Design review of the part built by this model. Coordinates are the model's own, in mm. A direction names the side the tool comes from. Give positions to 0.01 mm unless a question says otherwise; leave off trailing zeros. Loops run counter-clockwise (first coordinate to the right, second up) from the corner with the lowest first, then second, coordinate; pieces in that order, holes last.
from build123d import *
from build123d.topology import SkipClean

# Parameters (mm, degrees)
BOSS_EXTRUDE1_DEPTH      = 15
CHAMFER1_SIZE            = 3.2
LPATTERN1_COUNT          = 2
LPATTERN1_PITCH          = 41.5
SKETCH4_W                = 5.3
SKETCH4_H                = 12.8
CUT_EXTRUDE1_DEPTH       = 81.375680401
SKETCH5_W                = 26.8
SKETCH5_H                = 15.8
CUT_EXTRUDE2_DEPTH       = 3.5
CUT_EXTRUDE_THIN11_REACH = 81.437
SKETCH6_W                = 26
SKETCH6_H                = 1.6


with BuildPart() as part:
    # Sketch1 → Boss-Extrude1 (new, symmetric)
    with BuildSketch(Plane(origin=(0, 0, 0), x_dir=(0, 0, -1), z_dir=(1, 0, 0))):
        Polygon((0, 0), (12, 3), (23.32165913, 12.5), (31.5, 12.5), (39.819620609, 6), (74, 6), (77, 3.65614312), (77, -3.157724852), (70, -11.5), (16, -11.5), (13.31488118, -8.3), (4.2, -4.6), align=None)
        Polygon((16.321122645, 3.753956381), (24.122393645, 10.3), (30.742479251, 10.3), (39.121033004, 3.753956381), align=None, mode=Mode.SUBTRACT)
    extrude(amount=BOSS_EXTRUDE1_DEPTH, both=True)

    # Chamfer1
    chamfer1_edges = [part.edges().sort_by_distance(p)[0] for p in [
        (-15, -11.5, -43),
        (15, -11.5, -43),
    ]]
    chamfer(chamfer1_edges, length=CHAMFER1_SIZE)

    # Sketch2 → Cut-Revolve1 (revolve, cut)
    with BuildSketch(Plane.XY.offset(-22.3), mode=Mode.PRIVATE) as cut_revolve1_sk:
        Polygon((15, 2.4), (10.15, 2.4), (3.75, -4), (0, -4), (0, -6.7), (15, -6.7), align=None)
    cut_revolve1 = revolve(cut_revolve1_sk.sketch.rotate(Axis((0, -6.7, -22.3), (-1, 0, 0)), 90), axis=Axis((0, -6.7, -22.3), (-1, 0, 0)), mode=Mode.SUBTRACT)

    # Mirror1: Cut-Revolve1 across plane
    add(cut_revolve1.mirror(Plane(origin=(0, 0, 0), x_dir=(0, 0, 1), z_dir=(1, 0, 0))), mode=Mode.SUBTRACT)

    # LPattern1: Cut-Revolve1 ×2
    with Locations(*[(0, 0, -i * LPATTERN1_PITCH) for i in range(1, LPATTERN1_COUNT)]):
        add(cut_revolve1, mode=Mode.SUBTRACT)

    # Mirror2 copy 1 sketch → Mirror2 copy 1 (revolve, cut)
    with BuildSketch(Plane(origin=(0, 0, -63.8), x_dir=(-1, 0, 0), z_dir=(0, 0, 1))):
        Polygon((15, -2.4), (10.15, -2.4), (3.75, 4), (0, 4), (0, 6.7), (15, 6.7), align=None)
    revolve(axis=Axis((0, -6.7, -63.8), (-1, 0, 0)), mode=Mode.SUBTRACT)

    # Mirror2 copy 2 sketch → Mirror2 copy 2 (revolve, cut)
    with SkipClean():  # the faces are left unmerged after this step: merging them gives an invalid solid
        with BuildSketch(Plane(origin=(0, 0, -22.3), x_dir=(-1, 0, 0), z_dir=(0, 0, 1))):
            Polygon((15, -2.4), (10.15, -2.4), (3.75, 4), (0, 4), (0, 6.7), (15, 6.7), align=None)
        revolve(axis=Axis((0, -6.7, -22.3), (-1, 0, 0)), mode=Mode.SUBTRACT)

    # Sketch4 → Cut-Extrude1 (cut, through all)
    with BuildSketch(Plane(origin=(0, 6, 0), x_dir=(1, 0, 0), z_dir=(0, 1, 0))):
        with Locations((6.85, 48.219620609)):
            Rectangle(SKETCH4_W, SKETCH4_H)
    cut_extrude1 = extrude(amount=-CUT_EXTRUDE1_DEPTH, mode=Mode.SUBTRACT)

    # Mirror3: Cut-Extrude1 across plane
    add(cut_extrude1.mirror(Plane(origin=(0, 0, 0), x_dir=(0, 0, 1), z_dir=(1, 0, 0))), mode=Mode.SUBTRACT)

    # Sketch5 → Cut-Extrude2 (cut)
    with BuildSketch(Plane(origin=(0, 6, 0), x_dir=(1, 0, 0), z_dir=(0, 1, 0))):
        with Locations((0, 64.5)):
            Rectangle(SKETCH5_W, SKETCH5_H)
    extrude(amount=-CUT_EXTRUDE2_DEPTH, mode=Mode.SUBTRACT)

    # Sketch6 → Cut-Extrude-Thin11 (cut, up to next)
    with BuildSketch(Plane.XY, mode=Mode.PRIVATE) as cut_extrude_thin11_sk1:
        with Locations((0, 7.8)):
            Rectangle(SKETCH6_W, SKETCH6_H)
    cut_extrude_thin11_tool1 = extrude(cut_extrude_thin11_sk1.sketch, amount=-CUT_EXTRUDE_THIN11_REACH, mode=Mode.PRIVATE) & part.part
    # Sketch6 → Cut-Extrude-Thin11 (cut, up to next)
    with BuildSketch(Plane.XY, mode=Mode.PRIVATE) as cut_extrude_thin11_sk2:
        Polygon((13, 6), (13, 10.5), (-13, 10.5), (-13, 6), (-14.6, 6), (-14.6, 12.1), (14.6, 12.1), (14.6, 6), align=None)
    cut_extrude_thin11_tool2 = extrude(cut_extrude_thin11_sk2.sketch, amount=-CUT_EXTRUDE_THIN11_REACH, mode=Mode.PRIVATE) & part.part
    # Sketch6 → Cut-Extrude-Thin11 (cut, up to next)
    with BuildSketch(Plane.XY, mode=Mode.PRIVATE) as cut_extrude_thin11_sk3:
        with Locations((0, 9.3)):
            Rectangle(SKETCH6_W, SKETCH6_H)
    cut_extrude_thin11_tool3 = extrude(cut_extrude_thin11_sk3.sketch, amount=-CUT_EXTRUDE_THIN11_REACH, mode=Mode.PRIVATE) & part.part
    add(cut_extrude_thin11_tool1.solids().sort_by_distance((0, 7.8, 0))[0], mode=Mode.SUBTRACT)
    add(cut_extrude_thin11_tool2.solids().sort_by_distance((0, 10.581414, 0))[0], mode=Mode.SUBTRACT)
    add(cut_extrude_thin11_tool3.solids().sort_by_distance((0, 9.3, 0))[0], mode=Mode.SUBTRACT)


solid = part.part
Q1. Insertion check: pin 1 (1 mm diameter, centred on x = 1.5, y = 4, fed in from +Z); pin 2 (12 mm diameter, centred on x = 10, z = -41.5, fed in from +Y); pin 3 (6 mm diameter, centred on y = -6.7, z = -22.3, fed in from +X). Each pin has a flat end and moves straight along its axis. Give the tip position at first contact, or say it passes through.
Results:
pin 1: stops at z = -12.6
pin 2: stops at y = 9.37
pin 3: stops at x = 4.05
Q2. Draft analysis for pull direction X (two halves, no side actions). For faces 1 (the face through (0.2, -2.3, -2.1)), 2 (the face through (-4.77, -3.15, -64.92)), 3 (the face through (4.2, -3, -48)), state which applies: pulls with the +X half, pulls with the -X half, needs draft (parallel to the pull), parting line crosses it, or undercut.
Results:
face 1: needs draft
face 2: pulls with the -X half
face 3: undercut
Q3. Take a section at C-C (y = 8.5). Give the boundary of the cut face in (x, z), plus the area to 3 significant figures.
Results:
outline: (-15, -36.62) - (-14.6, -36.62) - (-14.6, -33.05) - (-15, -33.05) - close; (-15, -21.98) - (-14.6, -21.98) - (-14.6, -18.55) - (-15, -18.55) - close; (-13, -36.62) - (13, -36.62) - (13, -33.05) - (-13, -33.05) - close; (14.6, -36.62) - (15, -36.62) - (15, -33.05) - (14.6, -33.05) - close; (14.6, -21.98) - (15, -21.98) - (15, -18.55) - (14.6, -18.55) - close
area: 98.5 mm2
Q4. Tool access review of faces 4 (the face through (-4.2, -3, -48)), 5 (the face through (0, 12.1, -27)), 6 (the face through (13.4, 4, -64)), 7 (the face through (12.541, 2.176, -61.791)): name each direction out of +Z, -Z, +X, -X, +Y, -Y from which nothing blocks a thin tool from reaching the whole face with its end or side.
Results:
face 4: +Y, -Y
face 5: +Z, -Z
face 6: +Y
face 7: +X
Q5. Wall thickness on line 1 (X direction, y = -1.5, z = -45); line 2 (Z direction, x = -11.5, y = -7); line 3 (Z direction, x = 12.4, y = -6.7): over which ranges is each line inside the solid? List them lowest first.
Results:
line 1: x = -15 to -9.5, -4.2 to 4.2, 9.5 to 15
line 2: z = -73.78 to -72.9, -54.7 to -31.4, -13.2 to -10.11
line 3: z = -74.03 to -72.9, -54.7 to -31.4, -13.2 to -9.37
Q6. Take a section at B-B (x = -1.5). Give the number of separate pieces and of enclosed holes in the cut face, plus the area to 3 significant figures.
Results:
separate pieces: 2
enclosed holes: 2
area: 1,050 mm2
Q7. Take a section at A-A (z = -63.8). Give the boundary of the cut face in (x, y), plus the area to 3 significant figures.
Results:
outline: (-15, 2.4) - (-10.15, 2.4) - (-3.75, -4) - (3.75, -4) - (10.15, 2.4) - (15, 2.4) - (15, 6) - (13.4, 6) - (13.4, 2.5) - (-13.4, 2.5) - (-13.4, 6) - (-15, 6) - close; (-5.85, -11.5) - (5.85, -11.5) - (3.75, -9.4) - (-3.75, -9.4) - close
area: 123 mm2
